```python
from build123d import *

# Parameters (mm, degrees)
BOSS_EXTRUDE1_DEPTH      = 30
BOSS_EXTRUDE2_DEPTH      = 10
BOSS_EXTRUDE2_DEPTH_BACK = 10
SKETCH3_W                = 170
SKETCH3_H                = 100
CUT_EXTRUDE1_DEPTH       = 40
BOSS_EXTRUDE3_DEPTH      = 14


with BuildPart() as part:
    # Sketch1 → Boss-Extrude1 (new body)
    with BuildSketch(Plane(origin=(0, 0, 0), x_dir=(1, 0, 0), z_dir=(0, 1, 0))):
        with BuildLine():
            Line((0, 0), (305, 0))
            ThreePointArc((305, 0), (315.606601718, 4.393398282), (320, 15))
            Line((320, 15), (320, 85))
            ThreePointArc((320, 85), (315.606601718, 95.606601718), (305, 100))
            Line((305, 100), (2.5, 100))
            ThreePointArc((2.5, 100), (0.732233047, 99.267766953), (0, 97.5))
            Line((0, 97.5), (0, 0))
        make_face()
        with BuildLine():
            Line((20, 95), (300, 95))
            ThreePointArc((300, 95), (310.606601718, 90.606601718), (315, 80))
            Line((315, 80), (315, 20))
            ThreePointArc((315, 20), (310.606601718, 9.393398282), (300, 5))
            Line((300, 5), (20, 5))
            ThreePointArc((20, 5), (9.393398282, 9.393398282), (5, 20))
            Line((5, 20), (5, 80))
            ThreePointArc((5, 80), (9.393398282, 90.606601718), (20, 95))
        make_face(mode=Mode.SUBTRACT)
    extrude(amount=BOSS_EXTRUDE1_DEPTH)

    # Sketch2 → Boss-Extrude2 (add, two sides: drawn at the far end of the back side and taken through both)
    with BuildSketch(Plane.XY.offset(-50).offset(-BOSS_EXTRUDE2_DEPTH_BACK)):
        Polygon((315, 0), (315, 5), (312.5, 2.5), align=None)
    extrude(amount=BOSS_EXTRUDE2_DEPTH + BOSS_EXTRUDE2_DEPTH_BACK)

    # Sketch3 → Cut-Extrude1 (cut)
    with BuildSketch(Plane(origin=(0, 0, 0), x_dir=(1, 0, 0), z_dir=(0, 1, 0))):
        with Locations((85, 50)):
            Rectangle(SKETCH3_W, SKETCH3_H)
    extrude(amount=CUT_EXTRUDE1_DEPTH, mode=Mode.SUBTRACT)

    # Sketch4 → Boss-Extrude3 (add)
    with BuildSketch(Plane(origin=(170, 0, 0), x_dir=(0, 0, -1), z_dir=(1, 0, 0))):
        with BuildLine():
            ThreePointArc((98.4, 24), (98.136396103, 24.636396103), (97.5, 24.9))
            Line((97.5, 24.9), (97.5, 5.1))
            ThreePointArc((97.5, 5.1), (98.136396103, 5.363603897), (98.4, 6))
            Line((98.4, 6), (98.4, 24))
        make_face()
        with BuildLine():
            Line((97.5, 5.1), (97.5, 24.9))
            ThreePointArc((97.5, 24.9), (96.863603897, 24.636396103), (96.6, 24))
            Line((96.6, 24), (96.6, 6))
            ThreePointArc((96.6, 6), (96.863603897, 5.363603897), (97.5, 5.1))
        make_face()
        with BuildLine():
            ThreePointArc((3.4, 24), (3.136396103, 24.636396103), (2.5, 24.9))
            Line((2.5, 24.9), (2.5, 5.1))
            ThreePointArc((2.5, 5.1), (3.136396103, 5.363603897), (3.4, 6))
            Line((3.4, 6), (3.4, 24))
        make_face()
        with BuildLine():
            Line((2.5, 5.1), (2.5, 24.9))
            ThreePointArc((2.5, 24.9), (1.863603897, 24.636396103), (1.6, 24))
            Line((1.6, 24), (1.6, 6))
            ThreePointArc((1.6, 6), (1.863603897, 5.363603897), (2.5, 5.1))
        make_face()
    extrude(amount=-BOSS_EXTRUDE3_DEPTH)


solid = part.part
```
CAD build for the part. Positions are in the model's coordinates, mm. A direction names the side the tool comes from. Give positions to 0.01 mm unless a question says otherwise; leave off trailing zeros. Write each loop counter-clockwise with the first axis right and the second up, starting at its lowest first coordinate (ties: lowest second). Pieces come first, ordered by that corner, then holes. Notation, with made-up numbers: M 77,-14.75 L 125,-14.75 A10 cw 125,-8.75 Z; hole C 2,74.25 d6. An arc over 180 degrees is marked long. Return JSON: item names as keys, results as strings. Group by question number.
(1) Flat gauge pins, fed straight in: pin 1 Ø12 at (y, z) = (17, -34) entering from -X; pin 2 Ø4 at (x, y) = (163, 18) entering from -Z; pin 3 Ø4 at (x, y) = (163.5, 15.5) entering from +Z. Where does each tip first touch, or does it go through?
(2) Band-saw the part on A-A (x = 222.5). Give the cut face in (y, z), and give its area (3 significant figures).
(3) Band-saw the part on B-B (y = 15.75). Give the cut face in (x, z).
(4) Band-saw the part on D-D (z = -34). Give the cut face in (x, y).
(5) 3-axis set-ups, long thin cutter, end or side, ignore diameter. For faces 4 (the face through (163, 15, -98.4)), 5 (the face through (315, 15, -50)), 6 (the face through (310.72, 14.79, -9.51)): which of +Z, -Z, +X, -X, +Y, -Y reach the whole face in a straight line?
(6) Drill centre lines: L1, parallel to Z at x = 223, y = 7.25; L2, parallel to X at y = 6.5, z = -61.5; L3, parallel to Z at x = 313, y = 25.25. Where is each one in solid material? Low to high. Write a range as [from, to].
(7) Band-saw the part on C-C (x = 167). Give the cut face in (y, z), and give its area (3 significant figures).
(8) Mould opens along Z. For faces 1 (the face through (170, 15, -96)), 2 (the face through (237, 15, 0)), 3 (the face through (267, 0, -2)) say: pulls with the +Z half, pulls with the -Z half, needs draft (parallel to the pull), parting line crosses it, or undercut.
Entries:
{
 "1": {"pin 1": "stops at x = 315", "pin 2": "stops at z = -98.4", "pin 3": "stops at z = -1.6"},
 "2": {"outline": "M 0,-100 L 30,-100 L 30,-95 L 0,-95 Z; M 0,-5 L 30,-5 L 30,0 L 0,0 Z", "area": "300 mm^2"},
 "3": {"outline": "M 156,-98.4 L 170,-98.4 L 170,-100 L 305,-100 A15 ccw 320,-85 L 320,-15 A15 ccw 305,0 L 170,0 L 170,-1.6 L 156,-1.6 L 156,-3.4 L 170,-3.4 L 170,-5 L 300,-5 A15 cw 315,-20 L 315,-80 A15 cw 300,-95 L 170,-95 L 170,-96.6 L 156,-96.6 Z"},
 "4": {"outline": "M 315,0 L 320,0 L 320,30 L 315,30 Z"},
 "5": {"face 4": "-Z, -X, +Y, -Y", "face 5": "-X, +Y", "face 6": "-X, +Y, -Y"},
 "6": {"L1": "z = [-100, -95], [-5, 0]", "L2": "x = [315, 320]", "L3": "z = [-97.69, -87.48], [-12.52, -2.31]"},
 "7": {"outline": "M 6,-98.4 L 24,-98.4 A0.9 ccw 24,-96.6 L 6,-96.6 A0.9 ccw Z; M 6,-3.4 L 24,-3.4 A0.9 ccw 24,-1.6 L 6,-1.6 A0.9 ccw Z", "area": "69.9 mm^2"},
 "8": {"face 1": "undercut", "face 2": "pulls with the +Z half", "face 3": "needs draft"}
}
